Drawing for the job (mm, zero at the part's lowest x, y, z). A direction names the side the tool comes from. Give positions to 0.01 mm unless a question says otherwise; leave off trailing zeros. Order: outer loops, then holes, each group sorted by start corner. A loop starts at its lowest first (then second) coordinate and runs counter-clockwise, first axis right, second up. Notation, with made-up numbers: (44, 33) - (72, 33) arc R30 cw to (72, 61) - close; hole circle Ø3 at (-23, -15.75). An arc over 180 degrees is marked (long way). One line per item, written item: value.
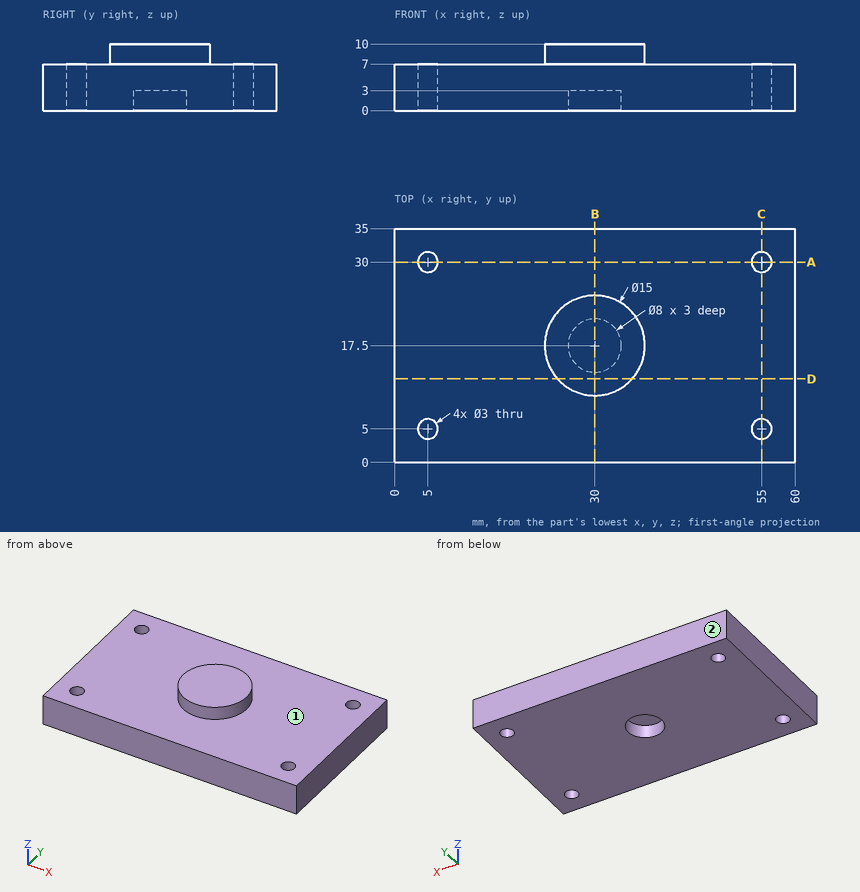
(1) Slice it at B-B, the plane x = 30. Give the cut face in (y, z), and give its area (3 significant figures).
Completed:
outline: (0, 0) - (13.5, 0) - (13.5, 3) - (21.5, 3) - (21.5, 0) - (35, 0) - (35, 7) - (25, 7) - (25, 10) - (10, 10) - (10, 7) - (0, 7) - close
area: 266 mm²
(2) 3-axis set-ups, long thin cutter, end or side, ignore diameter. For the marked faces 1 and 2: which of +Z, -Z, +X, -X, +Y, -Y reach the whole face in a straight line?
Completed:
face 1: +Z
face 2: +Z, -Z, +X, -X, +Y
(3) Drill centre lines: line 1 (Y direction, x = 55, z = 3.25); line 2 (Y direction, x = 56, z = 1.75); line 3 (Y direction, x = 30, z = 1.6). Where is each one in solid material? Low to high.
Completed:
line 1: 0 to 3.5, 6.5 to 28.5, 31.5 to 35
line 2: 0 to 3.88, 6.12 to 28.88, 31.12 to 35
line 3: 0 to 13.5, 21.5 to 35
(4) Slice it at C-C, the plane x = 55. Give the cut face in (y, z).
Completed:
outline: (0, 0) - (3.5, 0) - (3.5, 7) - (0, 7) - close; (6.5, 0) - (28.5, 0) - (28.5, 7) - (6.5, 7) - close; (31.5, 0) - (35, 0) - (35, 7) - (31.5, 7) - close
(5) Pin check, flat tips, straight feed: P1, Ø2.5, axis at x = 5, y = 5, coming from the -Z side; P2, Ø2.5, axis at x = 29.5, y = 19, coming from the -Z side; P3, Ø10, axis at x = 12, y = 23.5, coming from the +Z side. Stop position of each tip, or through.
Completed:
P1: through
P2: z = 3
P3: z = 7
(6) Slice it at D-D, the plane y = 12.5. Give the cut face in (x, z), and give its area (3 significant figures).
Completed:
outline: (0, 0) - (60, 0) - (60, 7) - (35.59, 7) - (35.59, 10) - (24.41, 10) - (24.41, 7) - (0, 7) - close
area: 454 mm²
(7) Slice it at A-A, the plane y = 30. Give the cut face in (x, z).
Completed:
outline: (0, 0) - (3.5, 0) - (3.5, 7) - (0, 7) - close; (6.5, 0) - (53.5, 0) - (53.5, 7) - (6.5, 7) - close; (56.5, 0) - (60, 0) - (60, 7) - (56.5, 7) - close
